from build123d import *

# Parameters (mm, degrees)
SKETCH1_R            = 11.065
EXTRUDE1_DEPTH       = 279.4
EXTRUDE1_2_DEPTH     = 279.4
EXTRUDE2_DEPTH       = 292.1
EXTRUDE2_DEPTH_BACK  = 114.3
SKETCH2_R            = 11.065
SKETCH3_R            = 11.065
EXTRUDE3_DEPTH       = 114.3
EXTRUDE5_DEPTH       = 413.085865385
EXTRUDE5_DEPTH_BACK  = 413.085865385
SKETCH5_W            = 50.8
SKETCH5_H            = 22.13
SKETCH7_R            = 11.065
SKETCH7_R_2          = 1.065
SKETCH7_W            = 28.83710894
SKETCH7_H            = 10
REVOLVE_THIN3_ANGLE  = 130
SKETCH10_R           = 11.065
EXTRUDE6_DEPTH       = 110.1
SKETCH11_W           = 5.1
SKETCH11_H           = 19.05
SKETCH11_H_2         = 15.156574232
EXTRUDE7_DEPTH       = 279.4
SKETCH12_W           = 234.581497294
SKETCH12_H           = 99.653287116
EXTRUDE8_DEPTH       = 5.1
EXTRUDE9_DEPTH       = 10
EXTRUDE9_DEPTH_BACK  = 10
SKETCH13_R           = 11.065
SKETCH13_R_2         = 10.565
EXTRUDE10_DEPTH      = 413.475527097
EXTRUDE10_DEPTH_BACK = 413.475527097
SKETCH14_R           = 10.565
SKETCH15_R           = 11.065
EXTRUDE11_DEPTH      = 28.4


with BuildPart() as part:
    # Sketch1 → Extrude1 (new body)
    with BuildSketch(Plane(origin=(0, 0, 0), x_dir=(1, 0, 0), z_dir=(0, 1, 0))):
        with Locations(Location((0, 0, 0), (0, 0, 270))):
            Circle(SKETCH1_R)
    extrude(amount=EXTRUDE1_DEPTH)



with BuildPart() as body_2:
    # Sketch1 → Extrude1 2 (new body)
    with BuildSketch(Plane(origin=(0, 0, 0), x_dir=(1, 0, 0), z_dir=(0, 1, 0))):
        with Locations(Location((279.4, 0, 0), (0, 0, 270))):
            Circle(SKETCH1_R)
    extrude(amount=EXTRUDE1_2_DEPTH)


with BuildPart() as part_1:
    add(part.part)

    add(body_2.part)  # Extrude2 merges body 2
    # Sketch2 → Extrude2 (add, two sides: drawn at the far end of the back side and taken through both)
    with BuildSketch(Plane(origin=(0, 0, 0), x_dir=(0, 0, -1), z_dir=(1, 0, 0)).offset(-EXTRUDE2_DEPTH_BACK)):
        with Locations((0, 279.4)):
            Circle(SKETCH2_R)
    extrude(amount=EXTRUDE2_DEPTH + EXTRUDE2_DEPTH_BACK)

    # Sketch3 → Extrude3 (add)
    with BuildSketch(Plane.ZY.offset(114.3)):
        with Locations((0, 177.8)):
            Circle(SKETCH3_R)
    extrude(amount=-EXTRUDE3_DEPTH)

    # Sketch5 → Extrude5 (cut, two sides: drawn at the far end of the back side and taken through both)
    with BuildSketch(Plane.XY.offset(-EXTRUDE5_DEPTH_BACK)):
        with Locations((-114.3, 177.8)):
            Rectangle(SKETCH5_W, SKETCH5_H)
    extrude(amount=EXTRUDE5_DEPTH + EXTRUDE5_DEPTH_BACK, mode=Mode.SUBTRACT)

    # Sketch7 → Revolve-Thin3 (revolve)
    # profile 1 of 2: a face of its own
    with BuildSketch(Plane.ZY.offset(88.9)):
        with Locations((0, 177.8)):
            Circle(SKETCH7_R)
        with Locations((0, 177.8)):
            Circle(SKETCH7_R_2, mode=Mode.SUBTRACT)
    # profile 2 of 2: a face of its own
    with BuildSketch(Plane.ZY.offset(88.9)):
        with Locations((14.41855447, 124.38)):
            Rectangle(SKETCH7_W, SKETCH7_H)
    revolve(axis=Axis((-88.9, 119.38, 0), (0, 0, 1)), revolution_arc=REVOLVE_THIN3_ANGLE)


with BuildPart() as revolve_thin3_kept_piece:
    # of the separate pieces the step leaves, the one the design keeps (revolve_thin3_pieces_kept)
    add(part_1.part.solids().sort_by_distance((0, 0, 11.065))[0])

    # Sketch10 → Extrude6 (add)
    with BuildSketch(Plane(origin=(-95.51451328, 113.829764346, 0), x_dir=(0.7660444431189746, 0.6427876096865435, 0), z_dir=(0.6427876096865435, -0.7660444431189746, 0))):
        with Locations(Location((-49.785366149, 0, 0), (0, 0, 180))):
            Circle(SKETCH10_R)
    extrude(amount=EXTRUDE6_DEPTH)

    # Sketch11 → Extrude7 (add)
    with BuildSketch(Plane(origin=(0, 0, 0), x_dir=(0, 0, -1), z_dir=(1, 0, 0))):
        with Locations((0, 177.8)):
            Rectangle(SKETCH11_W, SKETCH11_H)
        with Locations((0, 95.25)):
            Rectangle(SKETCH11_W, SKETCH11_H_2)
    extrude(amount=EXTRUDE7_DEPTH)

    # Sketch12 → Extrude8 (add)
    with BuildSketch(Plane.XY.offset(2.55)):
        with Locations((136.583327193, 137.498356442)):
            Rectangle(SKETCH12_W, SKETCH12_H)
    extrude(amount=EXTRUDE8_DEPTH)


with BuildPart() as extrude9_tool:
    # Sketch13 → Extrude9 (new, two sides: drawn at the far end of the back side and taken through both)
    with BuildSketch(Plane.XY.offset(-EXTRUDE9_DEPTH_BACK)):
        with Locations((279.4, 0)):
            Circle(SKETCH13_R)
        with Locations((279.4, 0)):
            Circle(SKETCH13_R_2, mode=Mode.SUBTRACT)
    extrude(amount=EXTRUDE9_DEPTH + EXTRUDE9_DEPTH_BACK)


with BuildPart() as revolve_thin3_kept_piece_1:
    add(revolve_thin3_kept_piece.part)


with BuildPart() as revolve_thin3_kept_piece_2:
    # Extrude9: joined with extrude9_tool
    add(revolve_thin3_kept_piece_1.part.fuse(extrude9_tool.part, tol=0.00001))

    # Sketch14 → Extrude10 (cut, two sides: drawn at the far end of the back side and taken through both)
    with BuildSketch(Plane(origin=(0, 0, -10), x_dir=(-1, 0, 0), z_dir=(0, 0, -1)).offset(-EXTRUDE10_DEPTH_BACK)):
        with Locations(Location((-279.4, 0, 0), (0, 0, 116.635810294))):
            Circle(SKETCH14_R)
    extrude(amount=EXTRUDE10_DEPTH + EXTRUDE10_DEPTH_BACK, mode=Mode.SUBTRACT)

    # Sketch15 → Extrude11 (add)
    with BuildSketch(Plane.XZ):
        with Locations(Location((0, 0, 0), (0, 0, 270))):
            Circle(SKETCH15_R)
    extrude(amount=EXTRUDE11_DEPTH)


solid = revolve_thin3_kept_piece_2.part
Source: CAD feature listing. Evaluate the final solid. Frame: model axes, mm. A direction names the side the tool comes from. Round coordinates to 2 decimals unless told otherwise and drop trailing zeros. Loops run counter-clockwise (first coordinate to the right, second up) from the corner with the lowest first, then second, coordinate; pieces in that order, holes last. Notation, with made-up numbers: (41.5, 0) - (67.5, 0) arc R23 cw to (67.5, 35) - close; hole circle Ø4 at (83.5, -15.5). An arc over 180 degrees is marked (long way). Write item = value, one per line. Start each with the question number.
Item 1: Section query B-B on y = 196.5. Output: boundary loops of the cut face in (x, z) (3 decimals).
Item 2: Material intervals for line 1 (Y direction, x = 83, z = -0.75) (3 decimals); line 2 (X direction, y = 0, z = 5.5) (3 decimals); line 3 (X direction, y = 25, z = 8.25), sorted ascending.
Item 3: First-contact query: pin 1 Ø10 at (y, z) = (69.5, 3) entering from +X (3 decimals); pin 2 Ø3 at (x, z) = (-102, 4.5) entering from +Y; pin 3 Ø16.5 at (x, y) = (95.5, 96) entering from -Z; pin 4 Ø5 at (x, z) = (144, 1) entering from +Y (3 decimals). Flat tips, straight axial feed; report the tip coordinate or a pass-through.
Item 4: Section query A-A on x = 99.5. Output: boundary loops of the cut face in (y, z) (3 decimals), plus the area to 3 significant figures.
Item 5: Reachability of faces 4 (the face through (86.06, 288.73, -5.95)), 5 (the face through (138, 178, -2.55)), 6 (the face through (15, 95, 2.55)), 7 (the face through (292.1, 280, 0)), 8 (the face through (135, 136, 2.55)) from +Z, -Z, +X, -X, +Y, -Y: full face, straight path, thin tool, end or side. Return the list, or none.
Item 6: Mould query, pull axis Y, two halves, no side actions, for faces 1 (the face through (138, 187.325, 2)), 2 (the face through (-114.3, 280, 0)), 3 (the face through (0, -28.4, 0)). Classes: released by +Y, released by -Y, zero draft, split by the parting line, or undercut.
Item 7: Section query C-C on x = -94.5. Count the separate pieces of the cut face and the enclosed holes in it, plus the area to 3 significant figures.
Results list:
q1.outline = circle Ø22.13 at (0, 0); circle Ø22.13 at (279.4, 0)
q2.line_1 = 87.672 to 102.828, 168.275 to 187.325, 268.36 to 290.44
q2.line_2 = -77.524 to -59.886, -9.601 to 9.601, 268.335 to 268.835, 289.965 to 290.465
q2.line_3 = -95.59 to -76.34, -7.37 to 7.37, 272.03 to 286.77
q3.pin_1 = 290.465
q3.pin_2 = 290.05
q3.pin_3 = -2.55
q3.pin_4 = 290.465
q4.outline = (87.672, -2.55) - (102.828, -2.55) - (102.828, 2.55) - (168.275, 2.55) - (168.275, -2.55) - (187.325, -2.55) - (187.325, 7.65) - (87.672, 7.65) - close; circle Ø22.13 at (279.4, 0)
q4.area = 1,070 mm²
q5.face_4 = none
q5.face_5 = -Z, -Y
q5.face_6 = +Z, -Y
q5.face_7 = +Z, -Z, +X, +Y, -Y
q5.face_8 = -Z
q6.face_1 = undercut
q6.face_2 = zero draft
q6.face_3 = released by -Y
q7.separate_pieces = 3
q7.enclosed_holes = 1
q7.area = 1,370 mm²
